from build123d import *

# Parameters (mm, degrees)
EXTRUDE2_DEPTH = 6.35


with BuildPart() as part:
    # Sketch1 → Extrude2 (new body)
    with BuildSketch(Plane.XY):
        Polygon((47.660264722, 0), (76.2, 0), (76.2, 6.35), (82.55, 6.35), (82.55, 0), (92.202, 0), (92.202, 6.35), (98.552, 6.35), (98.552, 0), (142.875, 0), (142.875, 41.275), (149.225, 41.275), (149.225, 0), (209.55, 0), (269.875, 0), (269.875, 41.275), (276.225, 41.275), (276.225, 0), (320.548, 0), (320.548, 6.35), (326.898, 6.35), (326.898, 0), (336.55, 0), (336.55, 6.35), (342.9, 6.35), (342.9, 0), (371.439735278, 0), (419.1, 82.55), (387.35, 82.55), (387.35, 88.9), (361.95, 88.9), (361.95, 82.55), (311.15, 82.55), (311.15, 88.9), (285.75, 88.9), (285.75, 82.55), (209.55, 82.55), (133.35, 82.55), (133.35, 88.9), (107.95, 88.9), (107.95, 82.55), (57.15, 82.55), (57.15, 88.9), (31.75, 88.9), (31.75, 82.55), (0, 82.55), align=None)
        with BuildLine():
            Line((170.020448202, 6.35), (249.079551798, 6.35))
            ThreePointArc((249.079551798, 6.35), (251.515549625, 8.170615133), (250.459410045, 11.022508199))
            Line((250.459410045, 11.022508199), (209.55, 37.493302934))
            Line((209.55, 37.493302934), (168.640589955, 11.022508199))
            ThreePointArc((168.640589955, 11.022508199), (167.584450375, 8.170615133), (170.020448202, 6.35))
        make_face(mode=Mode.SUBTRACT)
        with BuildLine():
            Line((155.575, 14.800584131), (155.575, 67.749415869))
            ThreePointArc((155.575, 67.749415869), (156.901171335, 69.98060837), (159.494858247, 69.881924069))
            Line((159.494858247, 69.881924069), (203.70555908, 41.275))
            Line((203.70555908, 41.275), (159.494858247, 12.668075931))
            ThreePointArc((159.494858247, 12.668075931), (156.901171335, 12.56939163), (155.575, 14.800584131))
        make_face(mode=Mode.SUBTRACT)
        with BuildLine():
            Line((170.020448202, 76.2), (249.079551798, 76.2))
            ThreePointArc((249.079551798, 76.2), (251.515549625, 74.379384867), (250.459410045, 71.527491801))
            Line((250.459410045, 71.527491801), (209.55, 45.056697066))
            Line((209.55, 45.056697066), (168.640589955, 71.527491801))
            ThreePointArc((168.640589955, 71.527491801), (167.584450375, 74.379384867), (170.020448202, 76.2))
        make_face(mode=Mode.SUBTRACT)
        with BuildLine():
            Line((136.525, 14.303625696), (136.525, 66.727414853))
            ThreePointArc((136.525, 66.727414853), (135.071559028, 69.023278411), (132.374614584, 68.691659953))
            Line((132.374614584, 68.691659953), (91.396300636, 35.095608642))
            Line((91.396300636, 35.095608642), (132.749939536, 12.084115469))
            ThreePointArc((132.749939536, 12.084115469), (135.272351238, 12.114030576), (136.525, 14.303625696))
        make_face(mode=Mode.SUBTRACT)
        with BuildLine():
            Line((104.902, 6.35), (120.207049127, 6.35))
            ThreePointArc((120.207049127, 6.35), (122.665621474, 8.252017233), (121.442109591, 11.109510228))
            Line((121.442109591, 11.109510228), (87.625811497, 29.926802573))
            ThreePointArc((87.625811497, 29.926802573), (86.163798888, 30.2371328), (84.780365617, 29.671537445))
            Line((84.780365617, 29.671537445), (61.828236325, 10.8542451))
            ThreePointArc((61.828236325, 10.8542451), (61.046887793, 8.034892566), (63.438621741, 6.35))
            Line((63.438621741, 6.35), (69.85, 6.35))
            Line((69.85, 6.35), (69.85, 12.7))
            Line((69.85, 12.7), (104.902, 12.7))
            Line((104.902, 12.7), (104.902, 6.35))
        make_face(mode=Mode.SUBTRACT)
        with BuildLine():
            Line((18.683371551, 62.889451217), (48.221461062, 11.727979426))
            ThreePointArc((48.221461062, 11.727979426), (49.965843374, 10.499123351), (52.031551003, 11.033734326))
            Line((52.031551003, 11.033734326), (77.262001053, 31.718906867))
            ThreePointArc((77.262001053, 31.718906867), (78.181456091, 33.910104112), (76.886676101, 35.902662194))
            Line((76.886676101, 35.902662194), (22.118136541, 66.378961445))
            ThreePointArc((22.118136541, 66.378961445), (19.07288135, 65.941246674), (18.683371551, 62.889451217))
        make_face(mode=Mode.SUBTRACT)
        with BuildLine():
            Line((27.316473501, 76.2), (124.41281719, 76.2))
            ThreePointArc((124.41281719, 76.2), (126.804551138, 74.515107434), (126.023202606, 71.6957549))
            Line((126.023202606, 71.6957549), (86.766032084, 39.510782213))
            ThreePointArc((86.766032084, 39.510782213), (85.382598814, 38.945186859), (83.920586204, 39.255517086))
            Line((83.920586204, 39.255517086), (26.081413037, 71.440489772))
            ThreePointArc((26.081413037, 71.440489772), (24.857901154, 74.297982767), (27.316473501, 76.2))
        make_face(mode=Mode.SUBTRACT)
        with BuildLine():
            Line((331.474188503, 29.926802573), (297.657890409, 11.109510228))
            ThreePointArc((297.657890409, 11.109510228), (296.434378526, 8.252017233), (298.892950873, 6.35))
            Line((298.892950873, 6.35), (314.198, 6.35))
            Line((314.198, 6.35), (314.198, 12.7))
            Line((314.198, 12.7), (349.25, 12.7))
            Line((349.25, 12.7), (349.25, 6.35))
            Line((349.25, 6.35), (355.661378259, 6.35))
            ThreePointArc((355.661378259, 6.35), (358.053112207, 8.034892566), (357.271763675, 10.8542451))
            Line((357.271763675, 10.8542451), (334.319634383, 29.671537445))
            ThreePointArc((334.319634383, 29.671537445), (332.936201112, 30.2371328), (331.474188503, 29.926802573))
        make_face(mode=Mode.SUBTRACT)
        with BuildLine():
            Line((327.703699364, 35.095608642), (286.350060464, 12.084115469))
            ThreePointArc((286.350060464, 12.084115469), (283.827648762, 12.114030576), (282.575, 14.303625696))
            Line((282.575, 14.303625696), (282.575, 66.727414853))
            ThreePointArc((282.575, 66.727414853), (284.028440972, 69.023278411), (286.725385416, 68.691659953))
            Line((286.725385416, 68.691659953), (327.703699364, 35.095608642))
        make_face(mode=Mode.SUBTRACT)
        with BuildLine():
            Line((341.837998947, 31.718906867), (367.068448997, 11.033734326))
            ThreePointArc((367.068448997, 11.033734326), (369.134156626, 10.499123351), (370.878538938, 11.727979426))
            Line((370.878538938, 11.727979426), (400.416628449, 62.889451217))
            ThreePointArc((400.416628449, 62.889451217), (400.02711865, 65.941246674), (396.981863459, 66.378961445))
            Line((396.981863459, 66.378961445), (342.213323899, 35.902662194))
            ThreePointArc((342.213323899, 35.902662194), (340.918543909, 33.910104112), (341.837998947, 31.718906867))
        make_face(mode=Mode.SUBTRACT)
        with BuildLine():
            Line((259.605141753, 69.881924069), (215.39444092, 41.275))
            Line((215.39444092, 41.275), (259.605141753, 12.668075931))
            ThreePointArc((259.605141753, 12.668075931), (262.198828665, 12.56939163), (263.525, 14.800584131))
            Line((263.525, 14.800584131), (263.525, 67.749415869))
            ThreePointArc((263.525, 67.749415869), (262.198828665, 69.98060837), (259.605141753, 69.881924069))
        make_face(mode=Mode.SUBTRACT)
        with BuildLine():
            Line((293.076797394, 71.6957549), (332.333967916, 39.510782213))
            ThreePointArc((332.333967916, 39.510782213), (333.717401186, 38.945186859), (335.179413796, 39.255517086))
            Line((335.179413796, 39.255517086), (393.018586963, 71.440489772))
            ThreePointArc((393.018586963, 71.440489772), (394.242098846, 74.297982767), (391.783526499, 76.2))
            Line((391.783526499, 76.2), (294.68718281, 76.2))
            ThreePointArc((294.68718281, 76.2), (292.295448862, 74.515107434), (293.076797394, 71.6957549))
        make_face(mode=Mode.SUBTRACT)
    extrude(amount=EXTRUDE2_DEPTH)


solid = part.part
The listing builds one solid part. Answer for the finished solid, in the listing's coordinates (mm). Give positions to 0.01 mm unless a question says otherwise; leave off trailing zeros. Write each loop counter-clockwise with the first axis right and the second up, starting at its lowest first coordinate (ties: lowest second). Pieces come first, ordered by that corner, then holes. Notation, with made-up numbers: (68.5, 86.25) -> (84.5, 86.25) arc R13 ccw to (84.5, 104.25) -> close; hole circle Ø1 at (-28.5, -29). An arc over 180 degrees is marked (long way). Use a Markdown table: item, result.
(1) Determine the mould class of faces 1 (the flat face through (209, 41, 6.35)), 2 (the flat face through (23.5, 41.85, 3.13)), 3 (the flat face through (363.69, 55.12, 3.13)) for opening direction Y: released by +Y, released by -Y, zero draft, split by the parting line, or undercut.
Return value:
| item | result |
|---|---|
| face 1 | zero draft |
| face 2 | released by -Y |
| face 3 | undercut |
(2) Find the intervals of material crossed by probe 1 along Y at (x, z) = (198, 4.5); probe 2 along Y at (x, z) = (84, 2.25); probe 3 along Y at (x, z) = (292.5, 1), in increasing order. Write a range as from..to.
Return value:
| item | result |
|---|---|
| probe 1 | 0..6.35, 30.02..37.58, 44.97..52.53, 76.2..82.55 |
| probe 2 | 0..12.7, 29.03..39.21, 76.2..82.55 |
| probe 3 | 0..15.51, 63.96..72.37, 74.95..88.9 |
(3) Section A-A, the plane x = 240 is taken. Determine the outline of the cut face in (y, z), then the cut area to 3 significant figures.
Return value:
| item | result |
|---|---|
| outline | (0, 0) -> (6.35, 0) -> (6.35, 6.35) -> (0, 6.35) -> close; (17.79, 0) -> (25.35, 0) -> (25.35, 6.35) -> (17.79, 6.35) -> close; (57.2, 0) -> (64.76, 0) -> (64.76, 6.35) -> (57.2, 6.35) -> close; (76.2, 0) -> (82.55, 0) -> (82.55, 6.35) -> (76.2, 6.35) -> close |
| area | 177 mm2 |
(4) Section B-B, the plane y = 22.5 is taken. Give the number of separate pieces and of enclosed holes in the cut face, then the cut area to 3 significant figures.
Return value:
| item | result |
|---|---|
| separate pieces | 12 |
| enclosed holes | 0 |
| area | 696 mm2 |
(5) Flat-ended cylindrical pins translate along their axes: P1, Ø3, axis at x = 94, z = 3, coming from the +Y side; P2, Ø1.9, axis at y = 2, z = 2.5, coming from the +X side; P3, Ø2, axis at y = 39, z = 3, coming from the +X side; P4, Ø12, axis at x = 150.5, y = 37, coming from the -Z side. Find the tip coordinate at first contact, or state that the pin passes through.
Return value:
| item | result |
|---|---|
| P1 | y = 82.55 |
| P2 | x = 373.14 |
| P3 | x = 394.53 |
| P4 | z = 0 |
